from build123d import *

# Parameters (mm, degrees)
SKETCH1_W                    = 406.4
SKETCH1_H                    = 58.7375
BASE_FLANGE1_DEPTH           = 1.51892
EDGE_FLANGE1_STRIP_W         = 9.88568
EDGE_FLANGE1_STRIP_H         = 1.51892
EDGE_FLANGE1_STRIP_CUT_DEPTH = 406.4
EDGE_FLANGE1_DEPTH           = 406.4
SKETCH10_W                   = 19.05
SKETCH10_H                   = 3.42392
CUT_EXTRUDE2_DEPTH           = 206.803161206
F_10_CLEARANCE_HOLE1_D       = 5.1054


# Sheet-metal steps are written as plain solids
with BuildPart() as part:
    # Sketch1 → Base-Flange1 (new body)
    with BuildSketch(Plane(origin=(0, 0, 0), x_dir=(0, 0, -1), z_dir=(1, 0, 0))):
        Rectangle(SKETCH1_W, SKETCH1_H)
    extrude(amount=-BASE_FLANGE1_DEPTH)

    # Edge-Flange1 strip (across the edge) → Edge-Flange1 strip cut (cut)
    with BuildSketch(Plane(origin=(0, 29.36875, -203.2), x_dir=(0, -1, 0), z_dir=(0, 0, 1))):
        with Locations((-1.51892, -0.75946)):
            Rectangle(EDGE_FLANGE1_STRIP_W, EDGE_FLANGE1_STRIP_H)
    extrude(amount=EDGE_FLANGE1_STRIP_CUT_DEPTH, mode=Mode.SUBTRACT)

    # Edge-Flange1 section (across the edge) → Edge-Flange1 (add)
    with BuildSketch(Plane(origin=(0, 29.36875, -203.2), x_dir=(0, -1, 0), z_dir=(0, 0, 1))):
        with BuildLine():
            Line((0, 1.905), (0, 12.7))
            Line((0, 12.7), (1.51892, 12.7))
            Line((1.51892, 12.7), (1.51892, 1.905))
            ThreePointArc((1.51892, 1.905), (2.076881582, 0.557961582), (3.42392, 0))
            Line((3.42392, 0), (3.42392, -1.51892))
            ThreePointArc((3.42392, -1.51892), (1.00284295, -0.51607705), (0, 1.905))
        make_face()
    extrude(amount=EDGE_FLANGE1_DEPTH)

    # Sketch10 → Cut-Extrude2 (cut, through all)
    with BuildSketch(Plane.ZY.offset(1.51892)):
        with Locations((-168.275, 27.65679)):
            Rectangle(SKETCH10_W, SKETCH10_H)
        with Locations((168.275, 27.65679)):
            Rectangle(SKETCH10_W, SKETCH10_H)
    extrude(amount=-CUT_EXTRUDE2_DEPTH, mode=Mode.SUBTRACT)

    # #10 Clearance Hole1 (through all)
    with Locations(Plane(origin=(0, 0, 0), x_dir=(0, 0, -1), z_dir=(1, 0, 0))):
        with Locations((-196.85, 2.38125), (196.85, -23.01875), (-196.85, -23.01875), (196.85, 2.38125)):
            Hole(F_10_CLEARANCE_HOLE1_D / 2)


solid = part.part
Design review of the part built by this model. Coordinates are the model's own, in mm. A direction names the side the tool comes from. Give positions to 0.01 mm unless a question says otherwise; leave off trailing zeros. Loops run counter-clockwise (first coordinate to the right, second up) from the corner with the lowest first, then second, coordinate; pieces in that order, holes last. Notation, with made-up numbers: (-23.5, 64.5) -> (29.5, 64.5) arc R33 ccw to (29.5, 102.5) -> close; hole circle Ø4 at (59.5, 78.5). An arc over 180 degrees is marked (long way). One line per question, with ' | ' between items. Start each with the question number.
(1) We need section B-B (z = -18.5). State the section outline as (x, y) points (3 decimals), and give its area (3 significant figures).
(2) We need section D-D (z = 170). State the section outline as (x, y) points, and give its area (3 significant figures).
(3) For faces 1 (the face through (7, 29.369, -191)), 2 (the face through (7, 27.85, 190)), list the 3-axis set-ups (+Z, -Z, +X, -X, +Y, -Y) from which the entire face can be reached by the end or side of a thin tool; tool diameter is ignored.
(4) For line 1 (Y direction, x = -0.55, z = -196.85); line 2 (Z direction, x = -0.5, y = -22); line 3 (Y direction, x = -0.35, z = 196.85), list the stretches that pass through material, from the lowest coordinate up.
(5) Insertion check: P1, Ø2, axis at y = -1.5, z = -33, coming from the +X side; P2, Ø5, axis at x = 8.5, z = 141, coming from the -Y side; P3, Ø0.8, axis at x = -0.5, z = -166, coming from the +Y side. Each pin has a flat end and moves straight along its axis. Give the tip position at first contact, or say it passes through.
(6) We need section C-C (y = -10.5). State the section outline as (x, z) points.
(7) Draft analysis for pull direction X (two halves, no side actions). For faces 3 (the face through (0, -1, 3)), 4 (the face through (-1.519, -1, 3)), 5 (the face through (7, 27.85, -191)), state which applies: +X half, -X half, draft (parallel to the pull), parting line (faces both ways), or undercut.
(8) We need section A-A (x = 8.25). State the section outline as (y, z) points, and give its area (3 significant figures).
The answers:
1) outline: (-1.519, -29.369) -> (0, -29.369) -> (0, 25.945) arc R1.905 cw to (1.905, 27.85) -> (12.7, 27.85) -> (12.7, 29.369) -> (1.905, 29.369) arc R3.424 ccw to (-1.519, 25.945) -> close | area: 107 mm^2
2) outline: (-1.52, -29.37) -> (0, -29.37) -> (0, 25.94) -> (-1.52, 25.94) -> close | area: 84.0 mm^2
3) face 1: +Z, -Z, +X, -X, +Y | face 2: +Z, -Z, +X, -Y
4) line 1: y = -29.37 to -25.57, -20.47 to -0.17, 4.93 to 28.33 | line 2: z = -203.2 to -199.19, -194.51 to 194.51, 199.19 to 203.2 | line 3: y = -29.37 to -25.57, -20.47 to -0.17, 4.93 to 28.52
5) P1: stops at x = 0 | P2: stops at y = 27.85 | P3: stops at y = 25.94
6) outline: (-1.52, -203.2) -> (0, -203.2) -> (0, 203.2) -> (-1.52, 203.2) -> close
7) face 3: +X half | face 4: -X half | face 5: draft
8) outline: (27.85, -203.2) -> (29.37, -203.2) -> (29.37, -177.8) -> (27.85, -177.8) -> close; (27.85, -158.75) -> (29.37, -158.75) -> (29.37, 158.75) -> (27.85, 158.75) -> close; (27.85, 177.8) -> (29.37, 177.8) -> (29.37, 203.2) -> (27.85, 203.2) -> close | area: 559 mm^2
